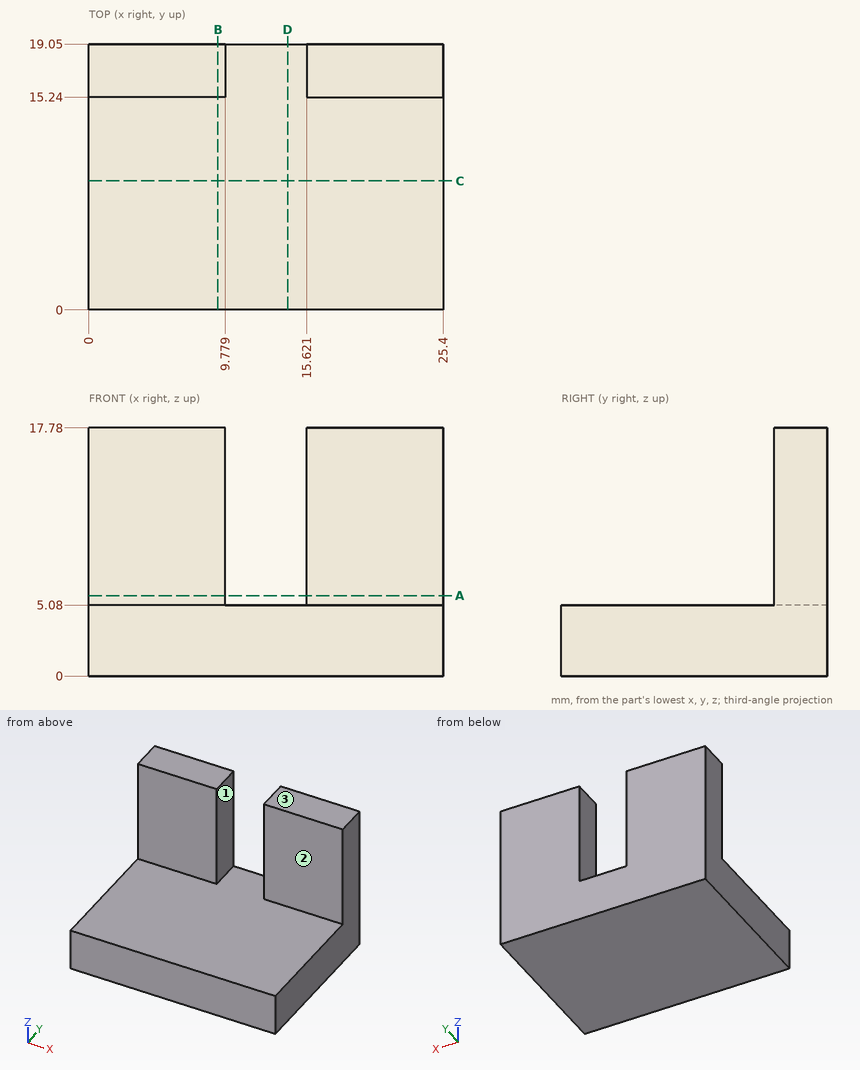
Drawing for the job (mm, zero at the part's lowest x, y, z). A direction names the side the tool comes from. Give positions to 0.01 mm unless a question says otherwise; leave off trailing zeros. Order: outer loops, then holes, each group sorted by start corner. A loop starts at its lowest first (then second) coordinate and runs counter-clockwise, first axis right, second up. Notation, with made-up numbers: M 66.5,-13 L 98.5,-13 A17 cw 98.5,-5 Z; hole C 86,75 d8. An arc over 180 degrees is marked long. Put each result on its own line as item: value. Start each with the question number.
(1) Saw through at A-A, the plane z = 5.75. Write the cut outline in (x, y), then the cut area to 3 significant figures.
(2) Saw through at D-D, the plane x = 14.25. Write the cut outline in (y, z), then the cut area to 3 significant figures.
(3) Saw through at C-C, the plane y = 9.25. Write the cut outline in (x, z).
(4) Flat gauge pins, fed straight in: pin 1 Ø5 at (x, z) = (22.5, 14) entering from -Y; pin 2 Ø6 at (x, y) = (7.5, 8.5) entering from +Z. Where does each tip first touch, or does it go through?
(5) Drill centre lines: line 1 along X through (y, z) = (15.75, 13.5); line 2 along Z through (x, y) = (10.75, 6.25); line 3 along Y through (x, z) = (16.75, 5.5). Where is each one in solid material? Low to high.
(6) Saw through at B-B, the plane x = 9.25. Write the cut outline in (y, z), then the cut area to 3 significant figures.
(7) Which spindle directions (+Z, -Z, +X, -X, +Y, -Y) get a long thin tool onto all of the face, cutting with end or side? Do the marked faces 1, 2 and 3. Say none if no direction does.
Check result:
1. outline: M 0,15.24 L 9.78,15.24 L 9.78,19.05 L 0,19.05 Z; M 15.62,15.24 L 25.4,15.24 L 25.4,19.05 L 15.62,19.05 Z
1. area: 74.5 mm2
2. outline: M 0,0 L 19.05,0 L 19.05,5.08 L 0,5.08 Z
2. area: 96.8 mm2
3. outline: M 0,0 L 25.4,0 L 25.4,5.08 L 0,5.08 Z
4. pin 1: stops at y = 15.24
4. pin 2: stops at z = 5.08
5. line 1: x = 0 to 9.78, 15.62 to 25.4
5. line 2: z = 0 to 5.08
5. line 3: y = 15.24 to 19.05
6. outline: M 0,0 L 19.05,0 L 19.05,17.78 L 15.24,17.78 L 15.24,5.08 L 0,5.08 Z
6. area: 145 mm2
7. face 1: +Z, +Y, -Y
7. face 2: +Z, +X, -X, -Y
7. face 3: +Z, +X, -X, +Y, -Y
